Could you check a few things on this drawing? It's one solid part, dimensions in mm from its lowest x, y, z. A direction names the side the tool comes from. Give positions to 0.01 mm unless a question says otherwise; leave off trailing zeros. Order: outer loops, then holes, each group sorted by start corner. A loop starts at its lowest first (then second) coordinate and runs counter-clockwise, first axis right, second up.
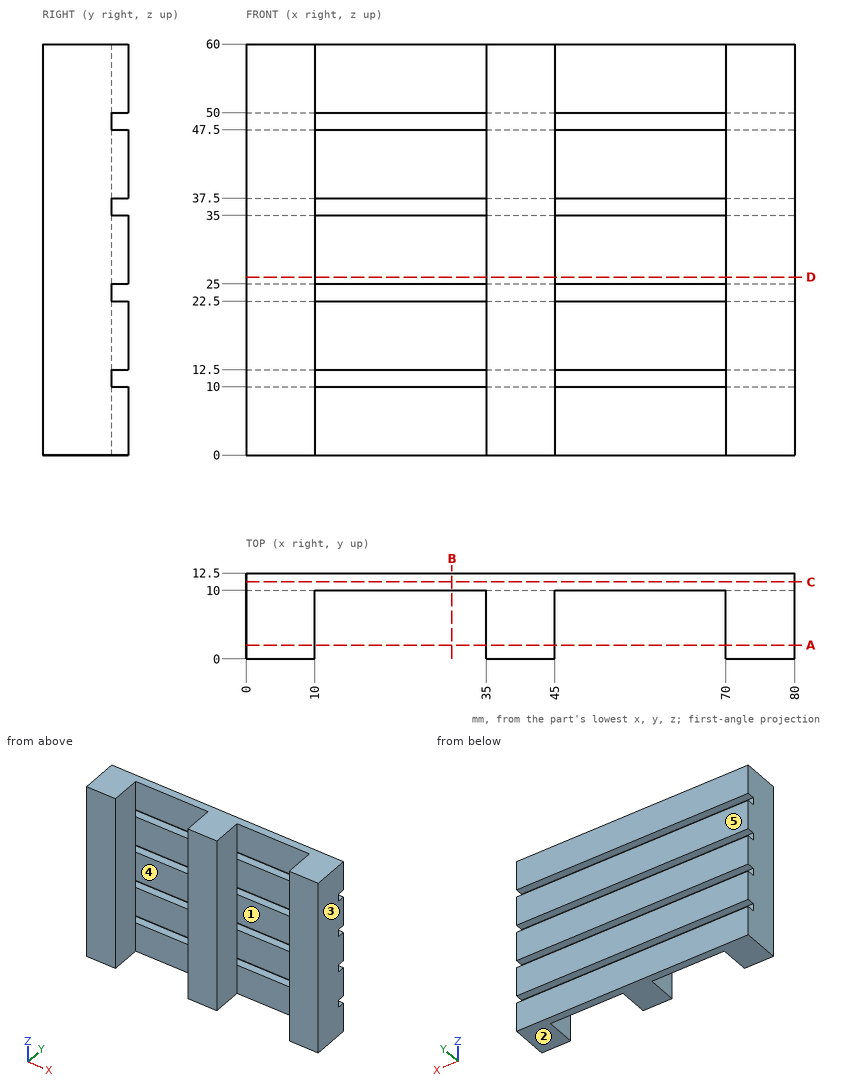
Q1. If we section it at A-A on y = 2: List the corners of the cut face in (x, z) for me, plus the area to 3 significant figures.
Filled sheet:
outline: (0, 0) - (10, 0) - (10, 60) - (0, 60) - close; (35, 0) - (45, 0) - (45, 60) - (35, 60) - close; (70, 0) - (80, 0) - (80, 60) - (70, 60) - close
area: 1,800 mm2
Q2. If we section it at C-C on y = 11.25: List the corners of the cut face in (x, z) for me, plus the area to 3 significant figures.
Filled sheet:
outline: (0, 0) - (80, 0) - (80, 10) - (0, 10) - close; (0, 12.5) - (80, 12.5) - (80, 22.5) - (0, 22.5) - close; (0, 25) - (80, 25) - (80, 35) - (0, 35) - close; (0, 37.5) - (80, 37.5) - (80, 47.5) - (0, 47.5) - close; (0, 50) - (80, 50) - (80, 60) - (0, 60) - close
area: 4,000 mm2
Q3. If we section it at B-B on x = 30: List the corners of the cut face in (y, z) for me, plus the area to 3 significant figures.
Filled sheet:
outline: (10, 0) - (12.5, 0) - (12.5, 10) - (10, 10) - close; (10, 12.5) - (12.5, 12.5) - (12.5, 22.5) - (10, 22.5) - close; (10, 25) - (12.5, 25) - (12.5, 35) - (10, 35) - close; (10, 37.5) - (12.5, 37.5) - (12.5, 47.5) - (10, 47.5) - close; (10, 50) - (12.5, 50) - (12.5, 60) - (10, 60) - close
area: 125 mm2
Q4. If we section it at D-D on z = 26: List the corners of the cut face in (x, y) for me, plus the area to 3 significant figures.
Filled sheet:
outline: (0, 0) - (10, 0) - (10, 10) - (35, 10) - (35, 0) - (45, 0) - (45, 10) - (70, 10) - (70, 0) - (80, 0) - (80, 12.5) - (0, 12.5) - close
area: 500 mm2
Q5. I'm going to push flat-ended pins straight in: P1, Ø0.8, axis at x = 4.5, z = 36.5, coming from the +Y side; P2, Ø2, axis at x = 68, z = 22.5, coming from the -Y side. Where does each tip first touch, or does it pass through?
Filled sheet:
P1: stops at y = 10
P2: stops at y = 10
Q6. Thinking about a two-plate mould opening in X: for the marked faces 1, 2 and 3, which applies, released by +X, released by -X, zero draft, split by the parting line, or undercut?
Filled sheet:
face 1: undercut
face 2: zero draft
face 3: released by +X
Q7. For the marked faces 4 and 5, which set-ups out of +Z, -Z, +X, -X, +Y, -Y let a thin tool reach every point of the face, with its end or its side?
Filled sheet:
face 4: +Z, -Z, -Y
face 5: +Z, -Z, +X, -X, +Y
Q8. I need wall thicknesses on L1, parallel to X at y = 5.25, z = 25; L2, parallel to Z at x = 10.5, y = 12; L3, parallel to Y at x = 56.5, z = 29. Which ranges of each line are inside material? Lowest first, please.
Filled sheet:
L1: x = 0 to 10, 35 to 45, 70 to 80
L2: z = 0 to 10, 12.5 to 22.5, 25 to 35, 37.5 to 47.5, 50 to 60
L3: y = 10 to 12.5
